Check sheet for the drawn part. Datum: minimum x, y, z corner. Units: mm. A direction names the side the tool comes from. Coordinates: 2 decimals unless noted, no trailing zeros. Order: outer loops, then holes, each group sorted by start corner. A loop starts at its lowest first (then second) coordinate and runs counter-clockwise, first axis right, second up. Notation, with made-up numbers: (10, 79) - (15, 79) arc R11 cw to (15, 85) - close; hole circle Ø11 at (83, -15.75). An arc over 180 degrees is marked (long way). Put each result on its own line as item: value.
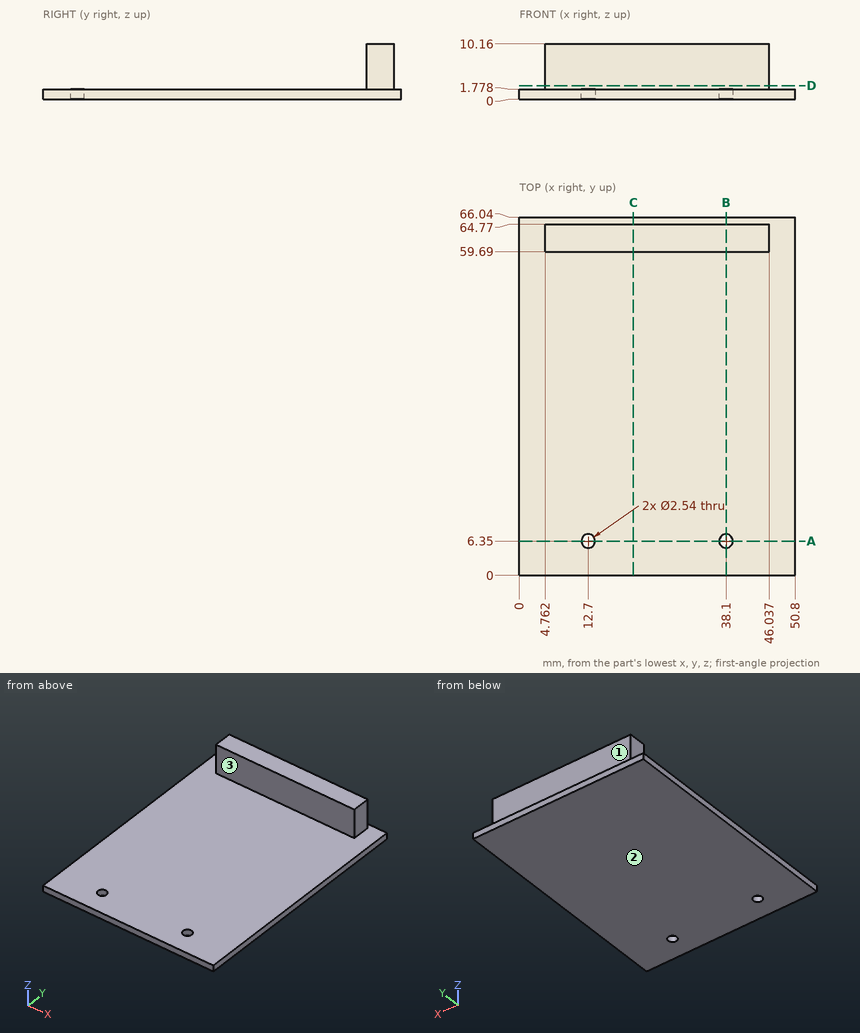
Q1. Section check A-A on y = 6.35. Record the boundary of the cut face in (x, z).
Answer block:
outline: (0, 0) - (11.43, 0) - (11.43, 1.78) - (0, 1.78) - close; (13.97, 0) - (36.83, 0) - (36.83, 1.78) - (13.97, 1.78) - close; (39.37, 0) - (50.8, 0) - (50.8, 1.78) - (39.37, 1.78) - close
Q2. Access from +Z, -Z, +X, -X, +Y, -Y to the whole of each face (thin tool, end or side, straight path). Record for the marked faces 1, 2 and 3.
Answer block:
face 1: +Z, +X, -X, +Y
face 2: -Z, +X, -X, +Y, -Y
face 3: +Z, +X, -X, -Y
Q3. Section check B-B on x = 38.1. Record the boundary of the cut face in (y, z).
Answer block:
outline: (0, 0) - (5.08, 0) - (5.08, 1.78) - (0, 1.78) - close; (7.62, 0) - (66.04, 0) - (66.04, 1.78) - (64.77, 1.78) - (64.77, 10.16) - (59.69, 10.16) - (59.69, 1.78) - (7.62, 1.78) - close
Q4. Depth check by flat-ended pin: pin 1 Ø5 at (x, y) = (6.5, 16.5) entering from +Z; pin 2 Ø1.5 at (y, z) = (62, 6.5) entering from -X; pin 3 Ø2 at (x, z) = (30.5, 8.5) entering from +Y; pin 4 Ø1.5 at (y, z) = (58.5, 8) entering from -X. Enter the tip coordinate at first touch or a pass-through.
Answer block:
pin 1: stops at z = 1.78
pin 2: stops at x = 4.76
pin 3: stops at y = 64.77
pin 4: passes through
Q5. Thickness scan on L1, parallel to Z at x = 5, y = 30; L2, parallel to Y at x = 43, z = 7. Record the ranges inside material, lowest first. Write a range as [from, to].
Answer block:
L1: z = [0, 1.78]
L2: y = [59.69, 64.77]
Q6. Section check D-D on z = 2.5. Record the boundary of the cut face in (x, y), then the cut area to 3 significant figures.
Answer block:
outline: (4.76, 59.69) - (46.04, 59.69) - (46.04, 64.77) - (4.76, 64.77) - close
area: 210 mm^2
Q7. Section check C-C on x = 21. Record the boundary of the cut face in (y, z).
Answer block:
outline: (0, 0) - (66.04, 0) - (66.04, 1.78) - (64.77, 1.78) - (64.77, 10.16) - (59.69, 10.16) - (59.69, 1.78) - (0, 1.78) - close
